Here's how the part is built. I have some questions about the finished solid (model axes, mm). Face numbers are marked on the shaded views. A direction names the side the tool comes from. Give positions to 0.01 mm unless a question says otherwise; leave off trailing zeros. Order: outer loops, then holes, each group sorted by start corner. A loop starts at its lowest first (then second) coordinate and runs counter-clockwise, first axis right, second up.
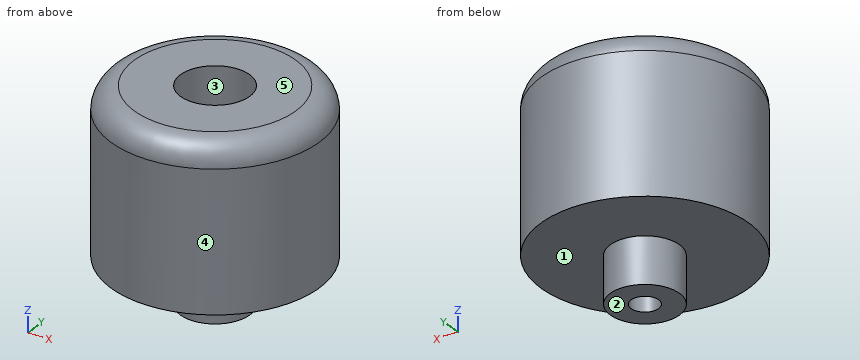
from build123d import *

# Parameters (mm, degrees)
F0_W   = 15
F0_H   = 15
F0_H_2 = 20
F0_W_2 = 4.5
F0_H_3 = 10
F2_R   = 5


with BuildPart() as f1:
    # F0 (on Front) → F1 (revolve)
    with BuildSketch(Plane.XZ):
        with Locations((15, 37.5)):
            Rectangle(F0_W, F0_H)
        with Locations((15, 20)):
            Rectangle(F0_W, F0_H_2)
        with Locations((5.25, 20)):
            Rectangle(F0_W_2, F0_H_2)
        with Locations((5.25, 5)):
            Rectangle(F0_W_2, F0_H_3)
    revolve(axis=Axis((0, 0, 22.5), (0, 0, 1)))

    # F2
    f2_edges = [f1.edges().sort_by_distance(p)[0] for p in [
        (-22.5, 0, 45),
    ]]
    fillet(f2_edges, radius=F2_R)


solid = f1.part
Q1. For the marked faces 1 and 2, which set-ups out of +Z, -Z, +X, -X, +Y, -Y let a thin tool reach every point of the face, with its end or its side?
Filled sheet:
face 1: -Z
face 2: -Z, +X, -X, +Y, -Y
Q2. If we section it at D-D on z = 33: List the corners of the cut face in (x, y) for me.
Filled sheet:
outline: circle Ø45 at (0, 0); hole circle Ø15 at (0, 0)
Q3. I'm going to push flat-ended pins straight in: P1, Ø12, axis at x = 0.5, z = 36, coming from the +Y side; P2, Ø1.5, axis at y = -15.5, z = 31, coming from the +X side; P3, Ø5.5, axis at x = 0, y = 0, coming from the -Z side; P4, Ø5, axis at x = -17.5, y = -16.5, coming from the -Z side. Where does each tip first touch, or does it pass through?
Filled sheet:
P1: stops at y = 22.5
P2: stops at x = 16.99
P3: passes through
P4: stops at z = 10
Q4. I need wall thicknesses on L1, parallel to Y at x = 0, z = 33.25; L2, parallel to Z at x = -12.5, y = 0.5; L3, parallel to Y at x = 0, z = 22.75. Which ranges of each line are inside material? Lowest first, please.
Filled sheet:
L1: y = -22.5 to -7.5, 7.5 to 22.5
L2: z = 10 to 45
L3: y = -22.5 to -3, 3 to 22.5
Q5. Thinking about a two-plate mould opening in X: for the marked faces 3, 4 and 5, which applies, released by +X, released by -X, zero draft, split by the parting line, or undercut?
Filled sheet:
face 3: undercut
face 4: split by the parting line
face 5: zero draft
Q6. If we section it at C-C on z = 9: List the corners of the cut face in (x, y) for me.
Filled sheet:
outline: circle Ø15 at (0, 0); hole circle Ø6 at (0, 0)
Q7. If we section it at A-A on x = 0: List the corners of the cut face in (y, z) for me, plus the area to 3 significant figures.
Filled sheet:
outline: (-22.5, 10) - (-7.5, 10) - (-7.5, 0) - (-3, 0) - (-3, 30) - (-7.5, 30) - (-7.5, 45) - (-17.5, 45) arc R5 ccw to (-22.5, 40) - close; (3, 0) - (7.5, 0) - (7.5, 10) - (22.5, 10) - (22.5, 40) arc R5 ccw to (17.5, 45) - (7.5, 45) - (7.5, 30) - (3, 30) - close
area: 1,310 mm2
